from build123d import *

# Parameters (mm, degrees)
BOSS_EXTRU_1_DEPTH      = 10
ESQUISSE2_R             = 1.025
ENL_V_MAT_EXTRU_1_DEPTH = 8
ENL_V_MAT_EXTRU_2_REACH = 130.997
ESQUISSE3_R             = 1.75
ESQUISSE4_R             = 3.5
ESQUISSE4_R_2           = 1.75
ENL_V_MAT_EXTRU_3_DEPTH = 4


with BuildPart() as part:
    # Esquisse1 → Boss.-Extru.1 (new body)
    with BuildSketch(Plane.XY):
        with BuildLine():
            Line((-12.5, -128), (12.5, -128))
            Line((12.5, -128), (10.205358779, -104.502873894))
            ThreePointArc((10.205358779, -104.502873894), (0, -105), (-10.205358779, -104.502873894))
            Line((-10.205358779, -104.502873894), (-12.5, -128))
        make_face()
    extrude(amount=BOSS_EXTRU_1_DEPTH)

    # Esquisse2 → Enlèv. mat.-Extru.1 (cut)
    with BuildSketch(Plane.XZ.offset(128)):
        with Locations((-4.75, 6)):
            Circle(ESQUISSE2_R)
        with Locations((4.75, 6)):
            Circle(ESQUISSE2_R)
    extrude(amount=-ENL_V_MAT_EXTRU_1_DEPTH, mode=Mode.SUBTRACT)

    # Esquisse3 → Enlèv. mat.-Extru.2 (cut, up to next)
    with BuildSketch(Plane.XY.offset(10), mode=Mode.PRIVATE) as enl_v_mat_extru_2_sk1:
        with Locations((-7.020582047, -114.785501819)):
            Circle(ESQUISSE3_R)
    enl_v_mat_extru_2_tool1 = extrude(enl_v_mat_extru_2_sk1.sketch, amount=-ENL_V_MAT_EXTRU_2_REACH, mode=Mode.PRIVATE) & part.part
    # Esquisse3 → Enlèv. mat.-Extru.2 (cut, up to next)
    with BuildSketch(Plane.XY.offset(10), mode=Mode.PRIVATE) as enl_v_mat_extru_2_sk2:
        with Locations((7.020582047, -114.785501819)):
            Circle(ESQUISSE3_R)
    enl_v_mat_extru_2_tool2 = extrude(enl_v_mat_extru_2_sk2.sketch, amount=-ENL_V_MAT_EXTRU_2_REACH, mode=Mode.PRIVATE) & part.part
    add(enl_v_mat_extru_2_tool1.solids().sort_by_distance((-7.020582, -114.785502, 10))[0], mode=Mode.SUBTRACT)
    add(enl_v_mat_extru_2_tool2.solids().sort_by_distance((7.020582, -114.785502, 10))[0], mode=Mode.SUBTRACT)

    # Esquisse4 → Enlèv. mat.-Extru.3 (cut)
    # profile 1 of 2: a face of its own
    with BuildSketch(Plane.XY.offset(10)):
        with Locations((7.020582047, -114.785501819)):
            Circle(ESQUISSE4_R)
        with Locations((7.020582047, -114.785501819)):
            Circle(ESQUISSE4_R_2, mode=Mode.SUBTRACT)
    # profile 2 of 2: a face of its own
    with BuildSketch(Plane.XY.offset(10)):
        with Locations((-7.020582047, -114.785501819)):
            Circle(ESQUISSE4_R)
    extrude(amount=-ENL_V_MAT_EXTRU_3_DEPTH, mode=Mode.SUBTRACT)


solid = part.part
Input: part model. Units: mm. Frame: model coordinates. A direction names the side the tool comes from. Coordinates: 2 decimals unless noted, no trailing zeros. Loops run counter-clockwise (first coordinate to the right, second up) from the corner with the lowest first, then second, coordinate; pieces in that order, holes last. Notation, with made-up numbers: (87.5, 76) -> (137.5, 76) arc R11 ccw to (137.5, 95) -> close; hole circle Ø10 at (74.25, -19). An arc over 180 degrees is marked (long way). One line per item, written item: value.
(1) Cut plane A-A (y = -113.5). Output: boundary loops of the cut face in (x, z).
Answer below:
outline: (-11.08, 0) -> (-8.21, 0) -> (-8.21, 6) -> (-10.28, 6) -> (-10.28, 10) -> (-11.08, 10) -> close; (-5.83, 0) -> (5.83, 0) -> (5.83, 6) -> (3.77, 6) -> (3.77, 10) -> (-3.77, 10) -> (-3.77, 6) -> (-5.83, 6) -> close; (8.21, 0) -> (11.08, 0) -> (11.08, 10) -> (10.28, 10) -> (10.28, 6) -> (8.21, 6) -> close
(2) Draft query along Z for faces 4 (the face through (-5.774, -124.056, 6.045)), 5 (the face through (-5, -120, 6)), 6 (the face through (-7.25, -113.05, 3.04)), 7 (the face through (0, -116, 10)). Return one class per face: pulls with the +Z half, pulls with the -Z half, needs draft (parallel to the pull), parting line crosses it, or undercut.
Answer below:
face 4: undercut
face 5: undercut
face 6: needs draft
face 7: pulls with the +Z half
(3) Ray query, line 1 along Z through (x, y) = (4.75, -124.5) (3 decimals); line 2 along X through (y, z) = (-124.25, 6.75); line 3 along X through (y, z) = (-114.5, 8.5). Return the intervals inside material, ascending.
Answer below:
line 1: z = 0 to 4.975, 7.025 to 10
line 2: x = -12.13 to -5.45, -4.05 to 4.05, 5.45 to 12.13
line 3: x = -11.18 to -10.51, -3.53 to 3.53, 10.51 to 11.18
(4) Set-up query: faces 1 (the face through (0, -116, 0)), 2 (the face through (-7.779, -118.202, 8.028)), 3 (the face through (5, -120, 6)). Return all of +Z, -Z, +X, -X, +Y, -Y with unobstructed straight access to the full face (end or side cutting, diameter ignored); none if empty.
Answer below:
face 1: -Z, +X, -X, +Y, -Y
face 2: +Z
face 3: -Y
(5) Cut plane D-D (y = -125). Output: boundary loops of the cut face in (x, z) (3 decimals), then the cut area to 3 significant figures.
Answer below:
outline: (-12.207, 0) -> (12.207, 0) -> (12.207, 10) -> (-12.207, 10) -> close; hole circle Ø2.05 at (-4.75, 6); hole circle Ø2.05 at (4.75, 6)
area: 238 mm2
(6) Cut plane B-B (x = 7.75). Output: boundary loops of the cut face in (y, z).
Answer below:
outline: (-128, 0) -> (-116.38, 0) -> (-116.38, 6) -> (-118.21, 6) -> (-118.21, 10) -> (-128, 10) -> close; (-113.19, 0) -> (-104.71, 0) -> (-104.71, 10) -> (-111.36, 10) -> (-111.36, 6) -> (-113.19, 6) -> close
(7) Pin query (flat end, axial travel): pin 1 Ø2 at (x, y) = (7, -116.5) entering from +Z; pin 2 Ø1.2 at (x, z) = (4.75, 6) entering from -Y; pin 3 Ø5 at (x, z) = (7, 2) entering from +Y; pin 4 Ø2 at (x, y) = (7.02, -114.79) entering from +Z. Return the tip coordinate at first contact, or that it passes through.
Answer below:
pin 1: stops at z = 6
pin 2: stops at y = -120
pin 3: stops at y = -104.57
pin 4: passes through
(8) Cut plane C-C (z = 6.5). Output: boundary loops of the cut face in (x, y), then the cut area to 3 significant figures.
Answer below:
outline: (-12.5, -128) -> (-5.64, -128) -> (-5.64, -120) -> (-3.86, -120) -> (-3.86, -128) -> (3.86, -128) -> (3.86, -120) -> (5.64, -120) -> (5.64, -128) -> (12.5, -128) -> (10.21, -104.5) arc R105 cw to (-10.21, -104.5) -> close; hole circle Ø7 at (-7.02, -114.79); hole circle Ø7 at (7.02, -114.79)
area: 421 mm2
